Autodesk Inventor part; units mm, degrees
ref_plane "YZ Plane" through (0, 0, 0) normal (1, 0, 0) x (0, 1, 0)
ref_plane "XZ Plane" through (0, 0, 0) normal (0, 1, 0) x (-1, 0, 0)
ref_plane "XY Plane" through (0, 0, 0) normal (0, 0, 1) x (1, 0, 0)
sketch "Sketch1" plane through (0, 0, 0) normal (0, 0, 1) x (1, 0, 0)
  line L0 (37.5, 0) -> (37.5, 30)
  line L1 (37.5, 30) -> (22.1407, 42)
  line L2 (22.1407, 42) -> (-22.1407, 42)
  line L3 (-22.1407, 42) -> (-37.5, 30)
  line L4 (-37.5, 30) -> (-37.5, 0)
  circle A0 centre (-28.678, 21) radius 3.5
  circle A1 centre (28.678, 21) radius 3.5
  circle A2 centre (-15.5, 36.5) radius 1.75
  circle A3 centre (15.5, 36.5) radius 1.75
  circle A4 centre (-15.5, 5.5) radius 1.75
  circle A5 centre (15.5, 5.5) radius 1.75
  circle A6 centre (0, 21) radius 11.5
  line L5 (-37.5, 0) -> (-25, 0)
  line L6 (-25, 0) -> (-25, 3.2)
  line L7 (-25, 3.2) -> (25, 3.2)
  line L8 (25, 3.2) -> (25, 0)
  line L9 (25, 0) -> (37.5, 0)
  point P0 (0, 0)
  point P1 (0, 42)
  point P2 (0, 0)
  dimension "d0" = 30
  dimension "d1" = 30
  dimension "d3" = 128
  dimension "d4" = 75
  dimension "d5" = 7
  dimension "d7" = 7
  dimension "d9" = 28.678
  dimension "d10" = 28.678
  dimension "d13" = 3.5
  dimension "d14" = 3.5
  dimension "d15" = 15.5
  dimension "d16" = 15.5
  dimension "d21" = 3.5
  dimension "d22" = 3.5
  dimension "d23" = 31
  dimension "d24" = 23
  dimension "d28" = 50
  dimension "d29" = 12.5
  dimension "d30" = 3.2
  dimension "d31" = 17.8
  dimension "d32" = 2.3
  dimension "d33" = 128
  dimension "d34" = 44.2814
  dimension "d35" = 12
  dimension "d36" = 12
  dimension "d37" = 42
extrude "Extrusion2" add sketch "Sketch1" along normal blind 6
fillet "Fillet2" radius 6 4 edges at (22.1407, 42, 3) (37.5, 30, 3) (-22.1407, 42, 3) (-37.5, 30, 3)
equation "\"d1\" = d0"
equation "\"d7\" = d5"
equation "\"d14\" = d13"
equation "\"d21\" = d13"
equation "\"d22\" = d13"
properties part number "Tope riel motor"
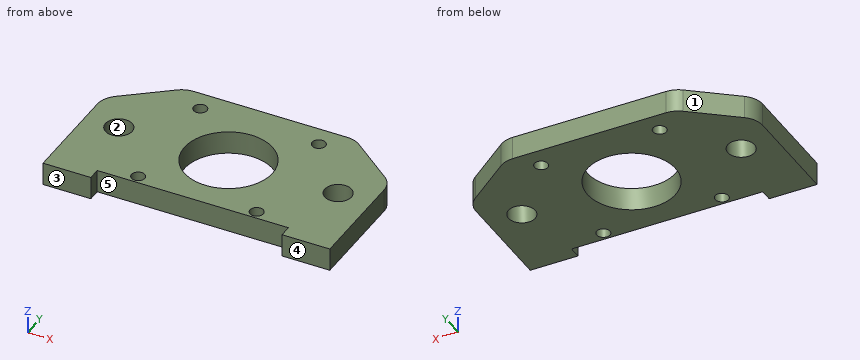
CAD build for the part. Positions are in the model's coordinates, mm. Face numbers are marked on the shaded views. A direction names the side the tool comes from. Round coordinates to 2 decimals unless told otherwise and drop trailing zeros. Loops run counter-clockwise (first coordinate to the right, second up) from the corner with the lowest first, then second, coordinate; pieces in that order, holes last.
(1) Drop flat-ended pins along their axis: pin 1 (9 mm diameter, centred on x = 28.678, y = 21, fed in from -Z); pin 2 (1.8 mm diameter, centred on x = 7, z = 2.5, fed in from -Y). Give the stop position or say it passes through.
(2) Cut at C-C (z = 4.6). Give the cut face in (x, y), plus the area to 3 significant figures.
(3) Which spindle directions (+Z, -Z, +X, -X, +Y, -Y) get a long thin tool onto all of the face, cutting with end or side? Do the marked faces 4 and 5. Say none if no direction does.
(4) Cut at A-A (y = 21). Give the cut face in (x, z).
(5) Wall check: line 1 along Y through (x, z) = (15.5, 2.8); line 2 along X through (y, z) = (4, 2.45); line 3 along X through (y, z) = (5, 5.4). Give the ranges that are in metal, low to high.
(6) Cut at D-D (x = 15.5). Give the cut face in (y, z).
(7) Cut at B-B (x = 0). Give the cut face in (y, z), plus the area to 3 significant figures.
(8) Two-plate mould, pull along Y, no slides. Class the marked faces 1, 2 and 3: +Y half, -Y half, draft (parallel to the pull), parting line (faces both ways), or undercut.
Findings below:
1. pin 1: stops at z = 0
1. pin 2: stops at y = 3.2
2. outline: (-37.5, 0) - (-25, 0) - (-25, 3.2) - (25, 3.2) - (25, 0) - (37.5, 0) - (37.5, 27.07) arc R6 ccw to (35.19, 31.8) - (23.77, 40.73) arc R6 ccw to (20.07, 42) - (-20.07, 42) arc R6 ccw to (-23.77, 40.73) - (-35.19, 31.8) arc R6 ccw to (-37.5, 27.07) - close; hole circle Ø7 at (-28.68, 21); hole circle Ø3.5 at (-15.5, 5.5); hole circle Ø3.5 at (-15.5, 36.5); hole circle Ø23 at (0, 21); hole circle Ø3.5 at (15.5, 5.5); hole circle Ø3.5 at (15.5, 36.5); hole circle Ø7 at (28.68, 21)
2. area: 2,270 mm2
3. face 4: +Z, -Z, +X, -X, -Y
3. face 5: +Z, -Z, -Y
4. outline: (-37.5, 0) - (-32.18, 0) - (-32.18, 6) - (-37.5, 6) - close; (-25.18, 0) - (-11.5, 0) - (-11.5, 6) - (-25.18, 6) - close; (11.5, 0) - (25.18, 0) - (25.18, 6) - (11.5, 6) - close; (32.18, 0) - (37.5, 0) - (37.5, 6) - (32.18, 6) - close
5. line 1: y = 3.2 to 3.75, 7.25 to 34.75, 38.25 to 42
5. line 2: x = -37.5 to -16.4, -14.6 to 14.6, 16.4 to 37.5
5. line 3: x = -37.5 to -17.18, -13.82 to 13.82, 17.18 to 37.5
6. outline: (3.2, 0) - (3.75, 0) - (3.75, 6) - (3.2, 6) - close; (7.25, 0) - (34.75, 0) - (34.75, 6) - (7.25, 6) - close; (38.25, 0) - (42, 0) - (42, 6) - (38.25, 6) - close
7. outline: (3.2, 0) - (9.5, 0) - (9.5, 6) - (3.2, 6) - close; (32.5, 0) - (42, 0) - (42, 6) - (32.5, 6) - close
7. area: 94.8 mm2
8. face 1: +Y half
8. face 2: undercut
8. face 3: -Y half
